```python
from build123d import *

# Parameters (mm, degrees)
EXTRUDE_1_DEPTH            = 10
HOLE_WIZARD_M4_D           = 4.5
HOLE_WIZARD_M4_CBORE_D     = 8
HOLE_WIZARD_M4_CBORE_DEPTH = 4
HOLE_WIZARD_1_4_201_D      = 5.1054
HOLE_WIZARD_3_8_161_D      = 7.9375
CUT_EXTRUDE_1_DEPTH        = 200.499373433
FILLET_1_R                 = 10
SKETCH_14_W                = 20.2
SKETCH_14_H                = 40
CUT_EXTRUDE_2_DEPTH        = 7
SKETCH_15_R                = 2
CUT_EXTRUDE_3_DEPTH        = 7
FILLET_2_R                 = 4


with BuildPart() as part:
    # Эскиз1 → Бобышка-Вытянуть1 (new body)
    with BuildSketch(Plane.XY):
        Polygon((0, 0), (60, 0), (60, -60), (60, -150), (60, -190), (0, -190), align=None)
    extrude(amount=EXTRUDE_1_DEPTH)

    # Цековка для винта с внутренним шестигранником M4 (through all)
    with Locations(Plane(origin=(-14.842707118, -41.655134189, 0), x_dir=(-1, 0, 0), z_dir=(0, 0, -1))):
        with Locations((-67.342707118, 36.655134189), (-52.342707118, 36.655134189), (-37.342707118, 36.655134189), (-22.342707118, 36.655134189)):
            CounterBoreHole(HOLE_WIZARD_M4_D / 2, HOLE_WIZARD_M4_CBORE_D / 2, HOLE_WIZARD_M4_CBORE_DEPTH)

    # Отверстие обработанное метчиком 1/4-201 (through all)
    with Locations(Plane(origin=(39.25, -175, 10), x_dir=(1, 0, 0), z_dir=(0, 0, 1))):
        with Locations((0, 0)):
            Hole(HOLE_WIZARD_1_4_201_D / 2)

    # Отверстие обработанное метчиком 3/8-161 (through all)
    with Locations(Plane(origin=(21, -175, 10), x_dir=(1, 0, 0), z_dir=(0, 0, 1))):
        with Locations((0, 0)):
            Hole(HOLE_WIZARD_3_8_161_D / 2)

    # Эскиз12 → Вырез-Вытянуть1 (cut, through all)
    with BuildSketch(Plane.XY.offset(10)):
        with BuildLine():
            Line((36.75, -175), (36.75, -70))
            ThreePointArc((36.75, -70), (39.25, -67.5), (41.75, -70))
            Line((41.75, -70), (41.75, -175))
            ThreePointArc((41.75, -175), (39.25, -177.5), (36.75, -175))
        make_face()
        with BuildLine():
            Line((18.5, -175), (18.5, -70))
            ThreePointArc((18.5, -70), (21, -67.5), (23.5, -70))
            Line((23.5, -70), (23.5, -175))
            ThreePointArc((23.5, -175), (21, -177.5), (18.5, -175))
        make_face()
    extrude(amount=-CUT_EXTRUDE_1_DEPTH, mode=Mode.SUBTRACT)

    # Скругление1
    fillet_1_edges = [part.edges().sort_by_distance(p)[0] for p in [
        (60, -190, 5),
        (0, -190, 5),
    ]]
    fillet(fillet_1_edges, radius=FILLET_1_R)

    # Эскиз14 → Вырез-Вытянуть2 (cut)
    with BuildSketch(Plane(origin=(0, 0, 0), x_dir=(-1, 0, 0), z_dir=(0, 0, -1))):
        with Locations((-30, -35)):
            Rectangle(SKETCH_14_W, SKETCH_14_H)
    extrude(amount=-CUT_EXTRUDE_2_DEPTH, mode=Mode.SUBTRACT)

    # Эскиз15 → Вырез-Вытянуть3 (cut)
    with BuildSketch(Plane(origin=(0, 0, 0), x_dir=(-1, 0, 0), z_dir=(0, 0, -1))):
        with Locations((-40.1, -55)):
            Circle(SKETCH_15_R)
        with Locations((-19.9, -55)):
            Circle(SKETCH_15_R)
    extrude(amount=-CUT_EXTRUDE_3_DEPTH, mode=Mode.SUBTRACT)

    # Скругление2
    fillet_2_edges = [part.edges().sort_by_distance(p)[0] for p in [
        (19.9, -15, 3.5),
        (40.1, -15, 3.5),
        (38.1, -55, 3.5),
        (40.1, -53, 3.5),
        (19.9, -53, 3.5),
        (21.9, -55, 3.5),
    ]]
    fillet(fillet_2_edges, radius=FILLET_2_R)


solid = part.part
```
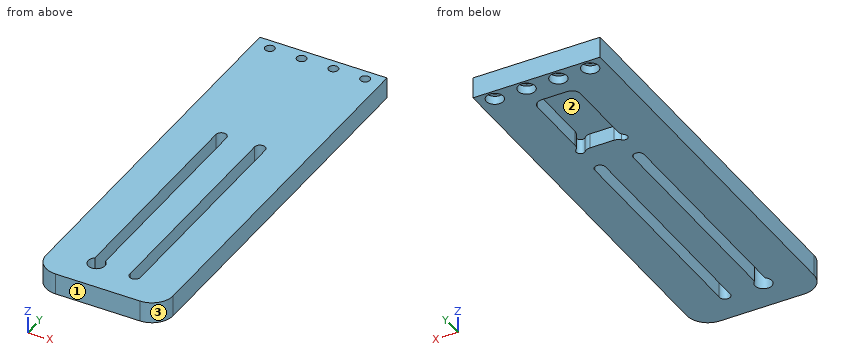
Work out the finished part from the listing and answer in its coordinate system (mm). Face numbers are marked on the shaded views. Coordinates: 2 decimals unless noted, no trailing zeros. Loops run counter-clockwise (first coordinate to the right, second up) from the corner with the lowest first, then second, coordinate; pieces in that order, holes last. Notation, with made-up numbers: (69.25, 35) -> (113.25, 35) arc R18 cw to (113.25, 56) -> close; hole circle Ø8 at (-8.5, -26.5). An arc over 180 degrees is marked (long way). Answer as CSV lines item,"result".
Q1. Each of these flat-tipped pins is pushed along its axis until it touches: pin 1 (2.5 mm diameter, centred on x = 39.5, y = -6.5, fed in from -Z); pin 2 (7.5 mm diameter, centred on x = 27.5, y = -32.5, fed in from -Z). Where does it stop, or does it pass through?
Findings:
pin 1,"stops at z = 4"
pin 2,"stops at z = 7"
Q2. For a pull along X with two mould halves and no side action, classify the marked faces 1, 2 and 3 as +X half, -X half, draft (parallel to the pull), parting line (faces both ways), or undercut.
Findings:
face 1,"draft"
face 2,"undercut"
face 3,"+X half"
Q3. The part is cut by section C-C on x = 52.5. Write down the section's boundary in (y, z).
Findings:
outline,"(-189.68, 0) -> (-9, 0) -> (-9, 4) -> (-7.25, 4) -> (-7.25, 10) -> (-189.68, 10) -> close; (-2.75, 4) -> (-1, 4) -> (-1, 0) -> (0, 0) -> (0, 10) -> (-2.75, 10) -> close"
Q4. The part is cut by section B-B on z = 8.5. Write down the section's boundary in (x, y), and give its area (3 significant figures).
Findings:
outline,"(0, -180) arc R10 ccw to (10, -190) -> (50, -190) arc R10 ccw to (60, -180) -> (60, 0) -> (0, 0) -> close; hole circle Ø4.5 at (7.5, -5); hole (18.5, -171.92) arc R3.97 ccw (long way) to (23.5, -171.92) -> (23.5, -70) arc R2.5 ccw to (18.5, -70) -> close; hole circle Ø4.5 at (22.5, -5); hole circle Ø4.5 at (37.5, -5); hole (36.75, -174.48) arc R2.55 ccw (long way) to (41.75, -174.48) -> (41.75, -70) arc R2.5 ccw to (36.75, -70) -> close; hole circle Ø4.5 at (52.5, -5)"
area,"10,200 mm²"
Q5. Find the intervals of material crossed by probe 1 along X at (y, z) = (-158, 4.5); probe 2 along X at (y, z) = (-175, 6.75); probe 3 along X at (y, z) = (-43.5, 3.25), in increasing order.
Findings:
probe 1,"x = 0 to 18.5, 23.5 to 36.75, 41.75 to 60"
probe 2,"x = 0 to 17.03, 24.97 to 36.7, 41.8 to 60"
probe 3,"x = 0 to 19.9, 40.1 to 60"
Q6. The part is cut by section A-A on y = -99.5. Write down the section's boundary in (x, z).
Findings:
outline,"(0, 0) -> (18.5, 0) -> (18.5, 10) -> (0, 10) -> close; (23.5, 0) -> (36.75, 0) -> (36.75, 10) -> (23.5, 10) -> close; (41.75, 0) -> (60, 0) -> (60, 10) -> (41.75, 10) -> close"
